```python
from build123d import *

# Parameters (mm, degrees)
F0_R     = 9.95
F1_DEPTH = 6


with BuildPart() as f1:
    # F0 (on Top) → F1 (new body)
    with BuildSketch(Plane.XY):
        with BuildLine():
            ThreePointArc((29.942197, 0), (34.641016, 20), (14.971099, 25.930703))
            ThreePointArc((14.971099, 25.930703), (0, 40), (-14.971099, 25.930703))
            ThreePointArc((-14.971099, 25.930703), (-34.641016, 20), (-29.942197, 0))
            ThreePointArc((-29.942197, 0), (-34.641016, -20), (-14.971099, -25.930703))
            ThreePointArc((-14.971099, -25.930703), (0, -40), (14.971099, -25.930703))
            ThreePointArc((14.971099, -25.930703), (34.641016, -20), (29.942197, 0))
        make_face()
        with Locations((0, -25)):
            Circle(F0_R, mode=Mode.SUBTRACT)
        with Locations((-21.650635, -12.5)):
            Circle(F0_R, mode=Mode.SUBTRACT)
        with Locations((21.650635, -12.5)):
            Circle(F0_R, mode=Mode.SUBTRACT)
        with Locations((-21.650635, 12.5)):
            Circle(F0_R, mode=Mode.SUBTRACT)
        with BuildLine():
            ThreePointArc((-5.5, 9.526279), (0, 11), (5.5, 9.526279))
            ThreePointArc((5.5, 9.526279), (9.526279, 5.5), (11, 0))
            ThreePointArc((11, 0), (9.526279, -5.5), (5.5, -9.526279))
            ThreePointArc((5.5, -9.526279), (0, -11), (-5.5, -9.526279))
            ThreePointArc((-5.5, -9.526279), (-9.526279, -5.5), (-11, 0))
            ThreePointArc((-11, 0), (-9.526279, 5.5), (-5.5, 9.526279))
        make_face(mode=Mode.SUBTRACT)
        with Locations((0, 25)):
            Circle(F0_R, mode=Mode.SUBTRACT)
        with Locations((21.650635, 12.5)):
            Circle(F0_R, mode=Mode.SUBTRACT)
    extrude(amount=F1_DEPTH)


solid = f1.part
```
For this review, take the finished solid that the model builds, in its own axes (mm). Coordinates: 2 decimals unless noted, no trailing zeros. Write each loop counter-clockwise with the first axis right and the second up, starting at its lowest first coordinate (ties: lowest second). Pieces come first, ordered by that corner, then holes.
(1) The part is to be moulded in two halves that separate along Y. For faces 1 (the face through (5.35, 33.39, 2.96)), 2 (the face through (8, -8, 6)), 3 (the face through (-34.48, 20.27, 2.96)), say which applies: +Y half, -Y half, draft (parallel to the pull), parting line (faces both ways), or undercut.
(2) Add section A-A on x = 0. Give the boundary of the cut face in (y, z), then the cut area to 3 significant figures.
(3) Add section B-B on y = 12.5. Give the boundary of the cut face in (x, z).
(4) Wall thickness on probe 1 along Y at (x, z) = (22, 0.8); probe 2 along Y at (x, z) = (0, 4.05); probe 3 along Y at (x, z) = (-19.5, 5.3): over which ranges is each line inside the solid? List them lowest first.
(5) Add section D-D on z = 4. Give the boundary of the cut face in (x, y).
(6) For pin 1 Ø12 at (x, y) = (21.65, 12.5) entering from +Z; pin 2 Ø2 at (x, z) = (22, 4) entering from +Y, all flat-tipped, find the tip position at first contact; note any pin that passes through.
(7) Add section C-C on y = -25. Give the boundary of the cut face in (x, z), then the cut area to 3 significant figures.
Answer sheet:
1. face 1: undercut
1. face 2: draft
1. face 3: undercut
2. outline: (-40, 0) - (-34.95, 0) - (-34.95, 6) - (-40, 6) - close; (-15.05, 0) - (-11, 0) - (-11, 6) - (-15.05, 6) - close; (11, 0) - (15.05, 0) - (15.05, 6) - (11, 6) - close; (34.95, 0) - (40, 0) - (40, 6) - (34.95, 6) - close
2. area: 109 mm2
3. outline: (-36.65, 0) - (-31.6, 0) - (-31.6, 6) - (-36.65, 6) - close; (-11.7, 0) - (11.7, 0) - (11.7, 6) - (-11.7, 6) - close; (31.6, 0) - (36.65, 0) - (36.65, 6) - (31.6, 6) - close
4. probe 1: y = -27.5 to -22.44, -2.56 to 2.56, 22.44 to 27.5
4. probe 2: y = -40 to -34.95, -15.05 to -11, 11 to 15.05, 34.95 to 40
4. probe 3: y = -27.35 to -22.21, -2.79 to 2.79, 22.21 to 27.35
5. outline: (-29.94, 0) arc R15 ccw to (-14.97, -25.93) arc R15 ccw to (14.97, -25.93) arc R15 ccw to (29.94, 0) arc R15 ccw to (14.97, 25.93) arc R15 ccw to (-14.97, 25.93) arc R15 ccw to start; hole circle Ø19.9 at (-21.65, -12.5); hole circle Ø19.9 at (-21.65, 12.5); hole (-11, 0) arc R11 ccw to (-5.5, -9.53) arc R11 ccw to (5.5, -9.53) arc R11 ccw to (11, 0) arc R11 ccw to (5.5, 9.53) arc R11 ccw to (-5.5, 9.53) arc R11 ccw to start; hole circle Ø19.9 at (0, -25); hole circle Ø19.9 at (0, 25); hole circle Ø19.9 at (21.65, -12.5); hole circle Ø19.9 at (21.65, 12.5)
6. pin 1: passes through
6. pin 2: stops at y = 27.5
7. outline: (-29.94, 0) - (-9.95, 0) - (-9.95, 6) - (-29.94, 6) - close; (9.95, 0) - (29.94, 0) - (29.94, 6) - (9.95, 6) - close
7. area: 240 mm2
